Answer from the drawing. Dimensions are ordinates in mm from the lowest x, y and z of the part. A direction names the side the tool comes from. Give positions to 0.01 mm unless a question says otherwise; leave off trailing zeros. Order: outer loops, then holes, each group sorted by start corner. A loop starts at its lowest first (then second) coordinate and runs counter-clockwise, first axis right, second up. Notation, with made-up numbers: (-20.75, -36) - (19.25, -36) arc R18 cw to (19.25, -26) - close; hole circle Ø11 at (25, 12.25). An arc over 180 degrees is marked (long way). Write each question's results on one line, items separated by ' | '.
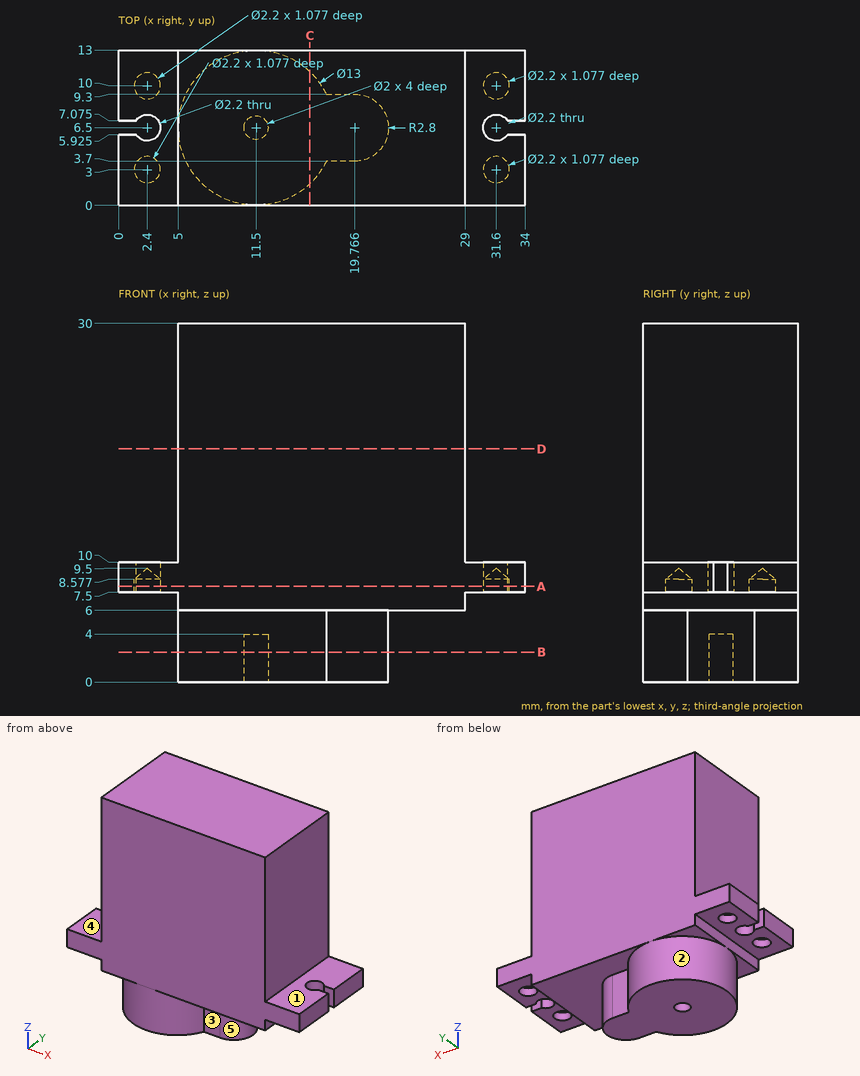
1. Straight lines are drawn through the part: line 1 (X direction, y = 10, z = 7.95); line 2 (Y direction, x = 2.4, z = 8.3); line 3 (Y direction, x = 2.4, z = 8.8) (1 decimal). For each, find the intervals that lie inside material, in ascending order. Write a range as [from, to].
Answer list:
line 1: [0, 1.3], [3.5, 30.5], [32.7, 34] | line 2: [0, 1.9], [4.1, 5.4], [7.6, 8.9], [11.1, 13] | line 3: [0, 2.2], [3.8, 5.4], [7.6, 9.2], [10.8, 13]
2. A tool of negligible diameter and unlimited length cuts with its end or side. For the marked faces 1, 2, 3, 4 and 5, from which of +Z, -Z, +X, -X, +Y, -Y can it reach the whole face along a straight path? Write none if from no direction.
Answer list:
face 1: +Z, +X, +Y, -Y | face 2: -Z | face 3: -Z, +X, -Y | face 4: +Z, -X, +Y, -Y | face 5: -Z, +X
3. A cutting plane is placed at D-D, the plane z = 19.5. Write down the section's boundary in (x, y), then the cut area to 3 significant figures.
Answer list:
outline: (5, 0) - (29, 0) - (29, 13) - (5, 13) - close | area: 312 mm^2
4. A cutting plane is placed at C-C, the plane x = 16. Write down the section's boundary in (y, z), then the cut area to 3 significant figures.
Answer list:
outline: (0, 6) - (1.81, 6) - (1.81, 0) - (11.19, 0) - (11.19, 6) - (13, 6) - (13, 30) - (0, 30) - close | area: 368 mm^2
5. Given P1, Ø4, axis at x = 32, y = 6.5, coming from the -Z side; P2, Ø4, axis at y = 9, z = 15, coming from the +X side; P3, Ø1.3, axis at x = 2.4, y = 6.5, coming from the +Z side; P4, Ø5, axis at y = 3, z = 20.5, coming from the -X side, each flat-ended and moving along its own axis, determine where each tip first touches the part or whether it passes through.
Answer list:
P1: z = 7.5 | P2: x = 29 | P3: through | P4: x = 5
6. A cutting plane is placed at B-B, the plane z = 2.5. Write down the section's boundary in (x, y), then the cut area to 3 significant figures.
Answer list:
outline: (17.37, 3.7) - (19.77, 3.7) arc R2.8 ccw to (19.77, 9.3) - (17.37, 9.3) arc R6.5 ccw (long way) to start; hole circle Ø2 at (11.5, 6.5) | area: 153 mm^2
7. A cutting plane is placed at A-A, the plane z = 8. Write down the section's boundary in (x, y) (1 decimal), then the cut area to 3 significant figures.
Answer list:
outline: (0, 0) - (34, 0) - (34, 5.9) - (32.5, 5.9) arc R1.1 cw (long way) to (32.5, 7.1) - (34, 7.1) - (34, 13) - (0, 13) - (0, 7.1) - (1.5, 7.1) arc R1.1 cw (long way) to (1.5, 5.9) - (0, 5.9) - close; hole circle Ø2.2 at (2.4, 3); hole circle Ø2.2 at (2.4, 10); hole circle Ø2.2 at (31.6, 3); hole circle Ø2.2 at (31.6, 10) | area: 416 mm^2
